Autodesk Inventor part; units mm, degrees
ref_plane "YZ Plane" through (0, 0, 0) normal (1, 0, 0) x (0, 1, 0)
ref_plane "XZ Plane" through (0, 0, 0) normal (0, 1, 0) x (-1, 0, 0)
ref_plane "XY Plane" through (0, 0, 0) normal (0, 0, 1) x (1, 0, 0)
sketch "スケッチ1" plane through (0, 0, 0) normal (0, 0, 1) x (1, 0, 0)
  line L0 (-16, 29) -> (16, 29)
  line L1 (16, 29) -> (16, -29)
  line L2 (16, -29) -> (-16, -29)
  line L3 (-16, -29) -> (-16, 29)
  point P0 (0, 0)
  point P1 (-16, 0)
  point P2 (0, -29)
  dimension "d0" = 32
  dimension "d1" = 58
extrude "押し出し1" add sketch "スケッチ1" along normal blind 28
fillet "フィレット1" radius 6 4 edges at (16, 0, 28) (-16, 0, 28) (-16, 0, 0) (16, 0, 0)
properties part number "AA-Cellx4"
Check sheet for the modelled part. Datum: model origin and axes. Units: mm. Round coordinates to 2 decimals unless told otherwise and drop trailing zeros. Loops run counter-clockwise (first coordinate to the right, second up) from the corner with the lowest first, then second, coordinate; pieces in that order, holes last.
1. Gauge pin test, flat end, axial feed: pin 1 Ø1.5 at (x, y) = (-1, -11) entering from -Z. Record the tip position at first contact, or that the pin passes through.
2. Scan lines: probe 1 along X at (y, z) = (25, 26); probe 2 along Z at (x, y) = (14, 12); probe 3 along X at (y, z) = (12.5, 25). Record each from-to range of solid material in increasing order.
3. Sectioned sample at A-A on y = -20.5. Record the boundary of the cut face in (x, z).
4. Sectioned sample at B-B on x = 12. Record the boundary of the cut face in (y, z), and give its area (3 significant figures).
Recorded:
1. pin 1: stops at z = 0
2. probe 1: x = -14.47 to 14.47
2. probe 2: z = 1.53 to 26.47
2. probe 3: x = -15.2 to 15.2
3. outline: (-16, 6) arc R6 ccw to (-10, 0) - (10, 0) arc R6 ccw to (16, 6) - (16, 22) arc R6 ccw to (10, 28) - (-10, 28) arc R6 ccw to (-16, 22) - close
4. outline: (-29, 0.34) - (29, 0.34) - (29, 27.66) - (-29, 27.66) - close
4. area: 1,580 mm2
